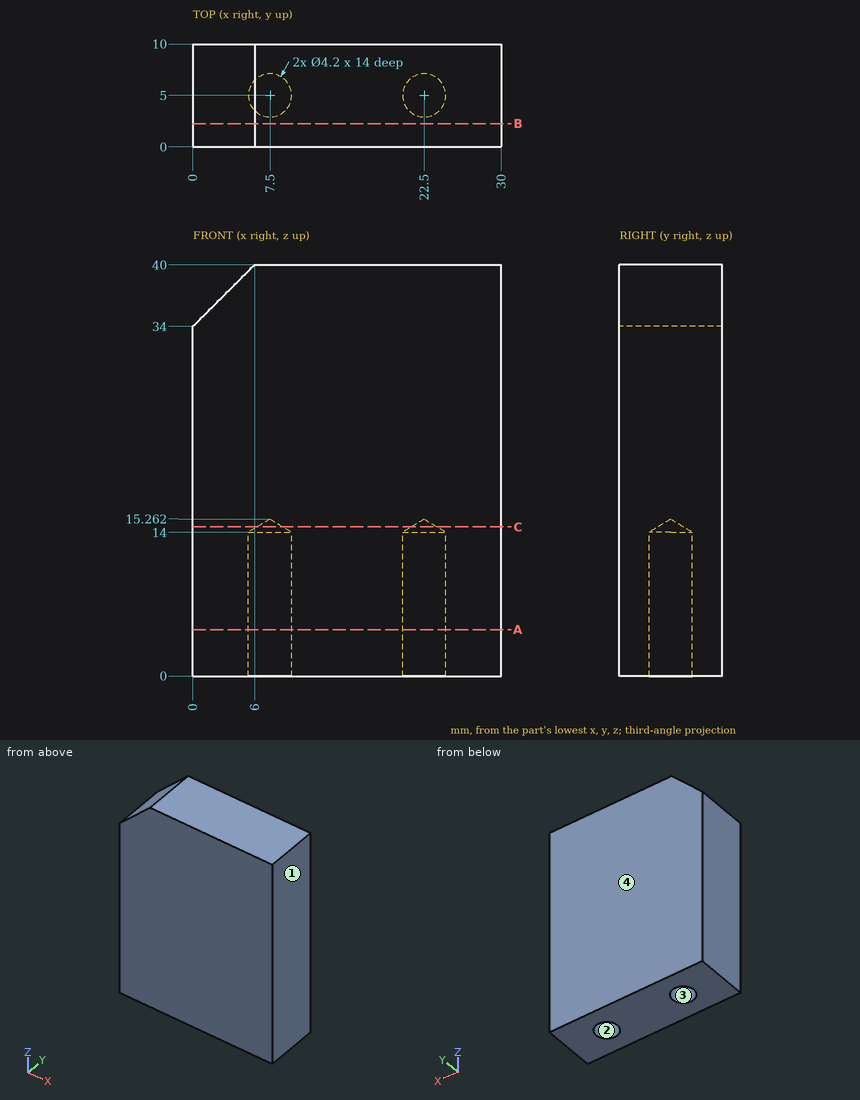
Here's the drawing with two shaded views (mm, measured from the low corner). I have some questions. Round coordinates to 2 decimals unless told otherwise and drop trailing zeros. Order: outer loops, then holes, each group sorted by start corner. A loop starts at its lowest first (then second) coordinate and runs counter-clockwise, first axis right, second up. Notation, with made-up numbers: (-0.5, 86) -> (30.5, 86) arc R24 ccw to (30.5, 101) -> close; hole circle Ø4 at (31, -5.5). An arc over 180 degrees is marked (long way). Use a Markdown table: item, result. Add a question column.
(1) I need wall thicknesses on line 1 along Y through (x, z) = (22.5, 4.25); line 2 along X through (y, z) = (4.5, 6); line 3 along X through (y, z) = (3, 37.5). Which ranges of each line are inside material? Lowest first, please.
(2) Suppose I cut it at B-B, the plane y = 2.25. Please give me the cut outline in (x, z), and give its area (3 significant figures).
(3) If we mould it in two halves opening along Y, with no side actions, what happens to the marked faces 1, 2, 3 and 4? For each: released by +Y, released by -Y, zero draft, split by the parting line, or undercut.
(4) Suppose I cut it at C-C, the plane z = 14.5. Please give me the cut outline in (x, y).
(5) Suppose I cut it at A-A, the plane z = 4.5. Please give me the cut outline in (x, y), and give its area (3 significant figures).
(6) For pin 1 Ø6 at (y, z) = (1.5, 21) entering from -X; pin 2 Ø3.5 at (x, y) = (7.5, 5) entering from -Z, each with a flat end and sliding along its axis, tell me the tip position at first contact or that it passes through.
Verdict:
| question | item | result |
|---|---|---|
| 1 | line 1 | 0 to 2.9, 7.1 to 10 |
| 1 | line 2 | 0 to 5.46, 9.54 to 20.46, 24.54 to 30 |
| 1 | line 3 | 3.5 to 30 |
| 2 | outline | (0, 0) -> (30, 0) -> (30, 40) -> (6, 40) -> (0, 34) -> close |
| 2 | area | 1,180 mm2 |
| 3 | face 1 | zero draft |
| 3 | face 2 | undercut |
| 3 | face 3 | undercut |
| 3 | face 4 | released by +Y |
| 4 | outline | (0, 0) -> (30, 0) -> (30, 10) -> (0, 10) -> close; hole circle Ø2.54 at (7.5, 5); hole circle Ø2.54 at (22.5, 5) |
| 5 | outline | (0, 0) -> (30, 0) -> (30, 10) -> (0, 10) -> close; hole circle Ø4.2 at (7.5, 5); hole circle Ø4.2 at (22.5, 5) |
| 5 | area | 272 mm2 |
| 6 | pin 1 | x = 0 |
| 6 | pin 2 | z = 14.21 |
